Check sheet for the modelled part. Datum: model origin and axes. Units: mm. A direction names the side the tool comes from. Round coordinates to 2 decimals unless told otherwise and drop trailing zeros. Write each loop counter-clockwise with the first axis right and the second up, starting at its lowest first coordinate (ties: lowest second). Pieces come first, ordered by that corner, then holes. Notation, with made-up numbers: (-32.75, 27.5) -> (-9.75, 27.5) arc R20 cw to (-9.75, 38.5) -> close; hole circle Ø2 at (51.5, -15). An arc over 180 degrees is marked (long way). One line per item, written item: value.
from build123d import *

# Parameters (mm, degrees)
BOSS_EXTRUDE1_DEPTH = 10
SKETCH8_R           = 4
CUT_EXTRUDE3_DEPTH  = 22
SKETCH14_R          = 3
CUT_EXTRUDE4_DEPTH  = 20


with BuildPart() as part:
    # Sketch1 → Boss-Extrude1 (new body)
    with BuildSketch(Plane(origin=(0, 0, 0), x_dir=(1, 0, 0), z_dir=(0, 1, 0))):
        with BuildLine():
            Line((12.93082957, 63.664368909), (12.93082957, -36.335631091))
            ThreePointArc((12.93082957, -36.335631091), (5.43082957, -43.835631091), (-2.06917043, -36.335631091))
            Line((-2.06917043, -36.335631091), (-2.06917043, 63.664368909))
            ThreePointArc((-2.06917043, 63.664368909), (5.43082957, 71.164368909), (12.93082957, 63.664368909))
        make_face()
    extrude(amount=BOSS_EXTRUDE1_DEPTH)

    # Sketch8 → Cut-Extrude3 (cut)
    with BuildSketch(Plane(origin=(0, 10, 0), x_dir=(1, 0, 0), z_dir=(0, 1, 0))):
        with Locations(Location((5.43082957, 63.664368909, 0), (0, 0, 270))):
            Circle(SKETCH8_R)
    extrude(amount=-CUT_EXTRUDE3_DEPTH, mode=Mode.SUBTRACT)

    # Sketch14 → Cut-Extrude4 (cut)
    with BuildSketch(Plane(origin=(0, 10, 0), x_dir=(1, 0, 0), z_dir=(0, 1, 0))):
        with Locations(Location((5.43082957, -36.335631091, 0), (0, 0, 270))):
            Circle(SKETCH14_R)
        Polygon((5.43082957, -21.527160564), (0.43082957, -21.527160564), (0.43082957, -26.531436495), (10.43082957, -26.531436495), (10.43082957, -21.527160564), align=None)
        Polygon((5.43082957, -6.509842668), (0.43082957, -6.509842668), (0.43082957, -11.527160564), (10.43082957, -11.527160564), (10.43082957, -6.509842668), align=None)
        Polygon((5.43082957, 8.538652281), (0.43082957, 8.538652281), (0.43082957, 3.51261249), (10.43082957, 3.51261249), (10.43082957, 8.538652281), align=None)
        Polygon((5.43082957, 23.544543967), (0.43082957, 23.544543967), (0.43082957, 18.538652281), (10.43082957, 18.538652281), (10.43082957, 23.544543967), align=None)
        Polygon((5.43082957, 38.56092778), (0.43082957, 38.56092778), (0.43082957, 33.544543967), (10.43082957, 33.544543967), (10.43082957, 38.56092778), align=None)
        Polygon((5.43082957, 53.568533881), (0.43082957, 53.568533881), (0.43082957, 48.56092778), (10.43082957, 48.56092778), (10.43082957, 53.568533881), align=None)
    extrude(amount=-CUT_EXTRUDE4_DEPTH, mode=Mode.SUBTRACT)


solid = part.part
Item 1: Material ranges on line 1 along X through (y, z) = (2.25, -21); line 2 along Z through (x, y) = (11, 3), recorded low to high.
Result set:
line 1: -2.07 to 0.43, 10.43 to 12.93
line 2: -68.69 to 41.36
Item 2: Sectioned sample at B-B (y = 3.25). State how many separate pieces and enclosed holes the cut face has, then the cut area to 3 significant figures.
Result set:
separate pieces: 1
enclosed holes: 8
area: 1,300 mm^2
Item 3: Sectioned sample at A-A (z = -21). Enter the section's corners in (x, y).
Result set:
outline: (-2.07, 0) -> (0.43, 0) -> (0.43, 10) -> (-2.07, 10) -> close; (10.43, 0) -> (12.93, 0) -> (12.93, 10) -> (10.43, 10) -> close
Item 4: Tool access check on faces 3 (the flat face through (10.431, 5, -21)), 4 (the flat face through (6, 10, -14)). Record the directions out of +Z, -Z, +X, -X, +Y, -Y that give a thin tool (end or side, any length) a straight path to the whole face; none if there is none.
Result set:
face 3: +Y, -Y
face 4: +Z, -Z, +X, -X, +Y
Item 5: Depth check by flat-ended pin: pin 1 (2 mm diameter, centred on x = 3, z = 24.5, fed in from +Y); pin 2 (5 mm diameter, centred on x = 8.5, y = 8.5, fed in from +Z); pin 3 (3 mm diameter, centred on x = 7.5, y = 3, fed in from -Z); pin 4 (4 mm diameter, centred on x = 0.5, y = 1.5, fed in from -Z). Enter the tip coordinate at first touch or a pass-through.
Result set:
pin 1: through
pin 2: z = 43.81
pin 3: z = -71.14
pin 4: z = -70.57
Item 6: Release check for a two-part mould opening along Z. For faces 1 (the flat face through (-2.069, 5, -13)), 2 (the flat face through (0.431, 5, -21)) record: pulls with the +Z half, pulls with the -Z half, needs draft (parallel to the pull), parting line crosses it, or undercut.
Result set:
face 1: needs draft
face 2: undercut
